from build123d import *

# Parameters (mm, degrees)
BASE_FLANGE1_DEPTH      = 56.388
EDGE_FLANGE2_DEPTH      = 58.5724
BREAK_CORNER3_START     = 1.706248663
BREAK_CORNER3_OUTLINE_W = 2
BREAK_CORNER3_OUTLINE_H = 81
BREAK_CORNER3_DEPTH     = 38.166088515
BREAK_CORNER4_START     = 1.706248663
BREAK_CORNER4_OUTLINE_W = 2
BREAK_CORNER4_OUTLINE_H = 81
BREAK_CORNER4_DEPTH     = 38.166088515
SKETCH21_R              = 8.89
SKETCH21_R_2            = 3.7211
SKETCH21_R_3            = 2.4892
SKETCH21_R_4            = 2.0701
CUT_EXTRUDE1_DEPTH      = 112.227490523
SKETCH22_R              = 3.429
CUT_EXTRUDE2_DEPTH      = 114.887063041
SKETCH23_R              = 2.0701
CUT_EXTRUDE3_DEPTH      = 114.887063041
FILLET1_R               = 6.35
CUT_EXTRUDE4_DEPTH      = 73.406


# Read off the part's stored shape, not the designer's step: Base-Flange1, Break-Corner3, Break-Corner4
# Sheet-metal steps are written as plain solids
with BuildPart() as part:
    # Base-Flange1 outline → Base-Flange1 (new body)
    with BuildSketch(Plane(origin=(0, 0, 0), x_dir=(1, 0, 0), z_dir=(0, 1, 0))):
        with BuildLine():
            Line((-66.77, 63.7032), (-66.77, 0))
            Line((-66.77, 0), (-64.77, 0))
            Line((-64.77, 0), (-64.77, 63.7032))
            ThreePointArc((-64.77, 63.7032), (-63.862382494, 65.894382494), (-61.6712, 66.802))
            Line((-61.6712, 66.802), (-3.0988, 66.802))
            ThreePointArc((-3.0988, 66.802), (-0.907617506, 65.894382494), (0, 63.7032))
            Line((0, 63.7032), (0, 0))
            Line((0, 0), (2, 0))
            Line((2, 0), (2, 63.7032))
            ThreePointArc((2, 63.7032), (0.506596056, 67.308596056), (-3.0988, 68.802))
            Line((-3.0988, 68.802), (-61.6712, 68.802))
            ThreePointArc((-61.6712, 68.802), (-65.276596056, 67.308596056), (-66.77, 63.7032))
        make_face()
    extrude(amount=BASE_FLANGE1_DEPTH)

    # Edge-Flange2 section (across the edge) → Edge-Flange2 (add)
    with BuildSketch(Plane(origin=(-61.6712, -5.08, -66.802), x_dir=(0, 1, 0), z_dir=(1, 0, 0))):
        with BuildLine():
            Line((0, 0.7366), (0, 66.58))
            Line((0, 66.58), (2, 66.58))
            Line((2, 66.58), (2, 0.7366))
            ThreePointArc((2, 0.7366), (2.215745145, 0.215745145), (2.7366, 0))
            Line((2.7366, 0), (5.08, 0))
            Line((5.08, 0), (5.08, -2))
            Line((5.08, -2), (2.7366, -2))
            ThreePointArc((2.7366, -2), (0.801531583, -1.198468417), (0, 0.7366))
        make_face()
    extrude(amount=EDGE_FLANGE2_DEPTH)

    # Break-Corner3 outline → Break-Corner3 (cut)
    with BuildSketch(Plane(origin=(0, 0, 0), x_dir=(1, 0, 0), z_dir=(0, 0.7071067811865476, 0.7071067811865476)).offset(BREAK_CORNER3_START)):
        with Locations((-65.77, 39.5)):
            Rectangle(BREAK_CORNER3_OUTLINE_W, BREAK_CORNER3_OUTLINE_H)
    extrude(amount=BREAK_CORNER3_DEPTH, mode=Mode.SUBTRACT)

    # Break-Corner4 outline → Break-Corner4 (cut)
    with BuildSketch(Plane(origin=(0, 0, 0), x_dir=(1, 0, 0), z_dir=(0, 0.7071067811865476, 0.7071067811865476)).offset(BREAK_CORNER4_START)):
        with Locations((1, 39.5)):
            Rectangle(BREAK_CORNER4_OUTLINE_W, BREAK_CORNER4_OUTLINE_H)
    extrude(amount=BREAK_CORNER4_DEPTH, mode=Mode.SUBTRACT)

    # Sketch21 → Cut-Extrude1 (cut, through all)
    with BuildSketch(Plane(origin=(0, 0, -68.802), x_dir=(-1, 0, 0), z_dir=(0, 0, -1))):
        with Locations((32.385, 28.194)):
            Circle(SKETCH21_R)
        with Locations((49.911, 45.72)):
            Circle(SKETCH21_R_2)
        with Locations((14.859, 10.668)):
            Circle(SKETCH21_R_2)
        with Locations((14.351, 46.228)):
            Circle(SKETCH21_R_3)
        with Locations((50.419, 10.16)):
            Circle(SKETCH21_R_3)
        with Locations((32.385, 42.672)):
            Circle(SKETCH21_R_4)
        with Locations((17.907, 28.194)):
            Circle(SKETCH21_R_4)
        with Locations(Location((32.385, 13.716, 0), (0, 0, 180))):
            Circle(SKETCH21_R_4)
        with Locations(Location((46.863, 28.194, 0), (0, 0, 180))):
            Circle(SKETCH21_R_4)
    extrude(amount=-CUT_EXTRUDE1_DEPTH, mode=Mode.SUBTRACT)

    # Sketch22 → Cut-Extrude2 (cut, through all)
    with BuildSketch(Plane.XZ.offset(5.08)):
        with Locations(Location((-48.238156, -57.372, 0), (0, 0, 270))):
            Circle(SKETCH22_R)
        with Locations(Location((-16.488156, -57.372, 0), (0, 0, 270))):
            Circle(SKETCH22_R)
        with Locations(Location((-32.363156, -57.372, 0), (0, 0, 270))):
            Circle(SKETCH22_R)
    extrude(amount=-CUT_EXTRUDE2_DEPTH, mode=Mode.SUBTRACT)

    # Sketch23 → Cut-Extrude3 (cut, through all)
    with BuildSketch(Plane.XZ.offset(5.08)):
        with Locations(Location((-41.888156, -37.23234, 0), (0, 0, 270))):
            Circle(SKETCH23_R)
        with Locations(Location((-41.888156, -11.83234, 0), (0, 0, 270))):
            Circle(SKETCH23_R)
        with Locations(Location((-22.838156, -37.23234, 0), (0, 0, 270))):
            Circle(SKETCH23_R)
        with Locations(Location((-22.838156, -11.83234, 0), (0, 0, 270))):
            Circle(SKETCH23_R)
    extrude(amount=-CUT_EXTRUDE3_DEPTH, mode=Mode.SUBTRACT)

    # Fillet1
    fillet1_edges = [part.edges().sort_by_distance(p)[0] for p in [
        (-61.6712, -4.08, -0.222),
        (-3.0988, -4.08, -0.222),
        (-65.77, 56.388, -53.975),
        (1, 56.388, -53.975),
    ]]
    fillet(fillet1_edges, radius=FILLET1_R)

    # Sketch24 → Cut-Extrude4 (cut)
    with BuildSketch(Plane.ZY.offset(66.77)):
        with BuildLine():
            Line((-0.499748663, 2.912748663), (0, 2.413))
            Line((0, 2.413), (1.847190311, 1.053295568))
            Line((1.847190311, 1.053295568), (0, 0))
            Line((0, 0), (-1.706248663, 0))
            ThreePointArc((-1.706248663, 0), (-0.129880446, 1.053295568), (-0.499748663, 2.912748663))
        make_face()
    extrude(amount=-CUT_EXTRUDE4_DEPTH, mode=Mode.SUBTRACT)


solid = part.part
Can you work these out from the model? Positions are in its coordinate system, mm. A direction names the side the tool comes from. Coordinates: 2 decimals unless noted, no trailing zeros. Order: outer loops, then holes, each group sorted by start corner. A loop starts at its lowest first (then second) coordinate and runs counter-clockwise, first axis right, second up. Notation, with made-up numbers: M 14.25,84 L 19.25,84 A27 ccw 19.25,121 Z; hole C 12,-12.75 d9. An arc over 180 degrees is marked long. Answer as CSV lines item,"result".
(1) Please list where these lines run through material, in increasing order: L1, parallel to X at y = 33, z = -52; L2, parallel to Z at x = -4.5, y = 53; L3, parallel to Y at x = -36, z = -17.5.
Geometry check:
L1,"-66.77 to -64.77, 0 to 2"
L2,"-68.8 to -66.8"
L3,"-5.08 to -3.08"
(2) On a 3-axis mill with a long thin cutter (end or side, diameter ignored), from which of +Z, -Z, +X, -X, +Y, -Y can I reach the whole of each face in a straight line? I mean faces 4 (the flat face through (-64.77, 22, -38)), 5 (the flat face through (-33, -5.08, -34)), 6 (the flat face through (-39, 20, -66.802)). Say none if no direction works.
Geometry check:
face 4,"+Z, +Y, -Y"
face 5,"+Z, -Z, +X, -X, -Y"
face 6,"+Z, +Y"
(3) If we mould it in two halves opening along Y, with no side actions, what happens to faces 1 (the flat face through (-33, -4, -0.222)), 2 (the cylindrical face through (-30.473, 14.509, -67.816)), 3 (the cylindrical face through (0.99, 1.03, -0.14))? For each: released by +Y, released by -Y, zero draft, split by the parting line, or undercut.
Geometry check:
face 1,"zero draft"
face 2,"undercut"
face 3,"split by the parting line"
(4) Suppose I cut it at C-C on y = 51.5. Please give me the cut outline in (x, z).
Geometry check:
outline,"M -66.77,-63.7 A5.1 ccw -61.67,-68.8 L -3.1,-68.8 A5.1 ccw 2,-63.7 L 2,-49.09 L 0,-49.09 L 0,-63.7 A3.1 cw -3.1,-66.8 L -61.67,-66.8 A3.1 cw -64.77,-63.7 L -64.77,-49.09 L -66.77,-49.09 Z"
(5) Suppose I cut it at D-D on z = -46. Please give me the cut outline in (x, y), plus the area to 3 significant figures.
Geometry check:
outline,"M -66.77,0 L -64.77,0 L -64.77,48.41 L -66.77,48.41 Z; M -61.67,-5.08 L -3.1,-5.08 L -3.1,-3.08 L -61.67,-3.08 Z; M 0,0 L 2,0 L 2,48.41 L 0,48.41 Z"
area,"311 mm^2"
(6) Suppose I cut it at A-A on z = -30.5. Please give me the cut outline in (x, y).
Geometry check:
outline,"M -66.77,0 L -64.77,0 L -64.77,32.91 L -66.77,32.91 Z; M -61.67,-5.08 L -3.1,-5.08 L -3.1,-3.08 L -61.67,-3.08 Z; M 0,0 L 2,0 L 2,32.91 L 0,32.91 Z"
(7) I'm going to push flat-ended pins straight in: pin 1 (1.5 mm diameter, centred on x = -0.5, z = -51.5, fed in from -Y); pin 2 (5.5 mm diameter, centred on x = -41.89, z = -37.23, fed in from +Y); pin 3 (0.6 mm diameter, centred on x = -28, y = -4, fed in from +Z). Where does each tip first touch, or does it pass through?
Geometry check:
pin 1,"y = 0"
pin 2,"y = -3.08"
pin 3,"z = -0.22"
(8) Suppose I cut it at B-B on z = -55. Please give me the cut outline in (x, y).
Geometry check:
outline,"M -66.77,0 L -64.77,0 L -64.77,56.18 L -66.77,56.18 Z; M -61.67,-5.08 L -50.71,-5.08 L -50.71,-3.08 L -61.67,-3.08 Z; M -45.76,-5.08 L -34.84,-5.08 L -34.84,-3.08 L -45.76,-3.08 Z; M -29.89,-5.08 L -18.96,-5.08 L -18.96,-3.08 L -29.89,-3.08 Z; M -14.01,-5.08 L -3.1,-5.08 L -3.1,-3.08 L -14.01,-3.08 Z; M 0,0 L 2,0 L 2,56.18 L 0,56.18 Z"
